from build123d import *

# Parameters (mm, degrees)
SKETCH1_R               = 48.5
SKETCH1_R_2             = 1.5
SKETCH1_W               = 5
SKETCH1_H               = 15
BOSS_EXTRUDE1_DEPTH     = 4
SKETCH1_4_W             = 5
SKETCH1_4_H             = 15
BOSS_EXTRUDE2_DEPTH     = 15
FILLET1_R               = 2
EXTRUDE_THIN1_DEPTH     = 11
SKETCH3_4_R             = 10.5
BOSS_EXTRUDE3_DEPTH     = 11
CUT_EXTRUDE2_DEPTH      = 11
SKETCH8_R               = 1.5
CUT_EXTRUDE3_DEPTH      = 9
SKETCH9_W               = 8
SKETCH9_H               = 4
CUT_EXTRUDE4_DEPTH      = 26
CUT_EXTRUDE4_DEPTH_BACK = 73


with BuildPart() as part:
    # Sketch1 → Boss-Extrude1 (new body)
    with BuildSketch(Plane(origin=(0, 0, 0), x_dir=(1, 0, 0), z_dir=(0, 1, 0))):
        Circle(SKETCH1_R)
        with Locations((7.5, 1.5)):
            Circle(SKETCH1_R_2, mode=Mode.SUBTRACT)
        with Locations((-7.5, 1.5)):
            Circle(SKETCH1_R_2, mode=Mode.SUBTRACT)
        with Locations((-21, -6)):
            Rectangle(SKETCH1_W, SKETCH1_H, mode=Mode.SUBTRACT)
    extrude(amount=BOSS_EXTRUDE1_DEPTH)

    # Sketch1<4> → Boss-Extrude2 (add)
    with BuildSketch(Plane(origin=(0, 0, 0), x_dir=(1, 0, 0), z_dir=(0, 1, 0))):
        with Locations((-21, -6)):
            Rectangle(SKETCH1_4_W, SKETCH1_4_H)
    extrude(amount=BOSS_EXTRUDE2_DEPTH)

    # Fillet1
    fillet1_edges = [part.edges().sort_by_distance(p)[0] for p in [
        (-21, 15, -1.5),
        (-21, 15, 13.5),
    ]]
    fillet(fillet1_edges, radius=FILLET1_R)

    # Sketch3 → Extrude-Thin1 (add, symmetric)
    with BuildSketch(Plane.XY.offset(-16)):
        with BuildLine():
            Line((-33.5, 0), (-33.5, 13.162084514))
            ThreePointArc((-33.5, 13.162084514), (-32.148724822, 19.384006302), (-28.338358569, 24.484924294))
            Line((-28.338358569, 24.484924294), (5.63016077, 54))
            ThreePointArc((5.63016077, 54), (37.663321214, 50.588409815), (31.952020166, 18.884413917))
            ThreePointArc((31.952020166, 18.884413917), (28.210951689, 15.065108917), (26.5, 10))
            Line((26.5, 10), (26.5, 0))
            Line((26.5, 0), (16.5, 0))
            Line((16.5, 0), (16.5, 10.429751474))
            ThreePointArc((16.5, 10.429751474), (19.537286112, 20.046443985), (26.546444335, 27.297484102))
            ThreePointArc((26.546444335, 27.297484102), (29.661699452, 44.590572773), (12.189066483, 46.451440147))
            Line((12.189066483, 46.451440147), (-21.779452856, 16.936364441))
            ThreePointArc((-21.779452856, 16.936364441), (-23.049574941, 15.236058444), (-23.5, 13.162084514))
            Line((-23.5, 13.162084514), (-23.5, 0))
            Line((-23.5, 0), (-33.5, 0))
        make_face()
    extrude(amount=EXTRUDE_THIN1_DEPTH, both=True)

    # Sketch3<4> → Boss-Extrude3 (add)
    with BuildSketch(Plane.XY.offset(-16)):
        with BuildLine():
            Line((-33.5, 0), (-33.5, 13.162084514))
            ThreePointArc((-33.5, 13.162084514), (-32.148724822, 19.384006302), (-28.338358569, 24.484924294))
            Line((-28.338358569, 24.484924294), (5.63016077, 54))
            ThreePointArc((5.63016077, 54), (37.663321214, 50.588409815), (31.952020166, 18.884413917))
            ThreePointArc((31.952020166, 18.884413917), (28.210951689, 15.065108917), (26.5, 10))
            Line((26.5, 10), (26.5, 0))
            Line((26.5, 0), (-33.5, 0))
        make_face()
        with Locations((20.059753337, 37.393168323)):
            Circle(SKETCH3_4_R, mode=Mode.SUBTRACT)
    extrude(amount=BOSS_EXTRUDE3_DEPTH)

    # Sketch5 → Cut-Extrude2 (cut)
    with BuildSketch(Plane(origin=(0, 0, -27), x_dir=(-1, 0, 0), z_dir=(0, 0, -1))):
        with BuildLine():
            Line((-16.5, 4), (25.5, 4))
            ThreePointArc((25.5, 4), (22.632303684, 20.469705569), (12.81364714, 34))
            Line((12.81364714, 34), (-7.597832484, 51.735432044))
            ThreePointArc((-7.597832484, 51.735432044), (-35.262834685, 48.789058703), (-30.330347417, 21.408334972))
            ThreePointArc((-30.330347417, 21.408334972), (-21.973239319, 13.849736754), (-16.5, 4))
        make_face()
    extrude(amount=-CUT_EXTRUDE2_DEPTH, mode=Mode.SUBTRACT)

    # Sketch8 → Cut-Extrude3 (cut)
    with BuildSketch(Plane(origin=(0, 0, -16), x_dir=(-1, 0, 0), z_dir=(0, 0, -1))):
        with Locations((-34.764358033, 43.204760253)):
            Circle(SKETCH8_R)
        with Locations((-28.336481936, 50.865204684)):
            Circle(SKETCH8_R)
        with Locations((8.433651334, 20.011399419)):
            Circle(SKETCH8_R)
        with Locations((2.005775237, 12.350954988)):
            Circle(SKETCH8_R)
        Polygon((-36.322950361, 36.680130765), (-22.181622948, 53.533108514), (9.992243663, 26.536028907), (-4.14908375, 9.683051158), align=None)
    extrude(amount=-CUT_EXTRUDE3_DEPTH, mode=Mode.SUBTRACT)

    # Sketch9 → Cut-Extrude4 (cut, two sides)
    with BuildSketch(Plane.ZY.offset(23.5)) as cut_extrude4_sk:
        with Locations((6, 9)):
            Rectangle(SKETCH9_W, SKETCH9_H)
    extrude(amount=CUT_EXTRUDE4_DEPTH, mode=Mode.SUBTRACT)
    extrude(cut_extrude4_sk.sketch, amount=-CUT_EXTRUDE4_DEPTH_BACK, mode=Mode.SUBTRACT)


solid = part.part
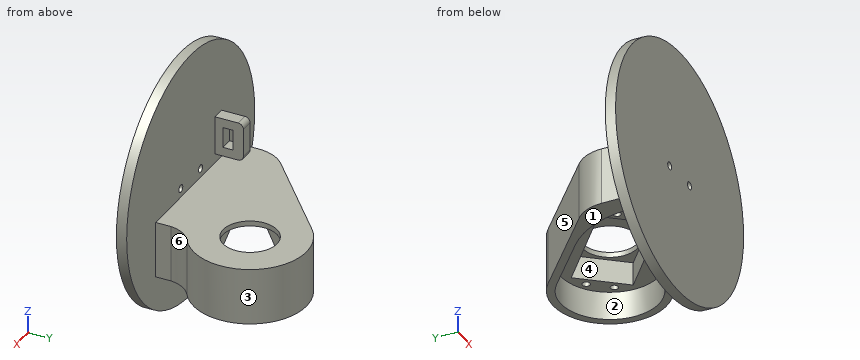
Could you check a few things on this model? Use its own coordinates, in mm. Face numbers are marked on the shaded views. A direction names the side the tool comes from. Give positions to 0.01 mm unless a question says otherwise; leave off trailing zeros. Order: outer loops, then holes, each group sorted by start corner. A loop starts at its lowest first (then second) coordinate and runs counter-clockwise, first axis right, second up. Notation, with made-up numbers: (33.25, 62.5) -> (49.25, 62.5) arc R13 cw to (49.25, 81.5) -> close; hole circle Ø1 at (68.5, -33.5). An arc over 180 degrees is marked (long way). Return JSON: item names as keys, results as strings.
1. Imagine slicing it at A-A on z = -23.5. List the corners of the cut face in (x, y) for me, then the cut area to 3 significant figures.
Answer list:
{"outline": "(-42.43, 0) -> (42.43, 0) -> (42.43, 4) -> (26.5, 4) -> (26.5, 10) arc R12 cw to (31.95, 18.88) arc R22 ccw (long way) to (5.63, 54) -> (-28.34, 24.48) arc R15 ccw to (-33.5, 13.16) -> (-33.5, 4) -> (-42.43, 4) -> close; hole (-25.5, 4) -> (16.5, 4) arc R34.47 cw to (30.33, 21.41) arc R19 ccw (long way) to (7.6, 51.74) -> (-12.81, 34) arc R37.03 ccw to start", "area": "965 mm2"}
2. Imagine slicing it at C-C on z = 40.5. List the corners of the cut face in (x, y) for me.
Answer list:
{"outline": "(-26.68, 0) -> (26.68, 0) -> (26.68, 4) -> (-26.68, 4) -> close"}
3. For pin 1 Ø5 at (x, z) = (-29, -1.5) entering from +Y; pin 2 Ø0.9 at (x, y) = (-2.5, 13) entering from -Z; pin 3 Ø12 at (y, z) = (13, 5) entering from +X, each with a flat end and sliding along its axis, tell me the tip position at first contact or that it passes through.
Answer list:
{"pin 1": "stops at y = 4", "pin 2": "stops at z = -7", "pin 3": "stops at x = -18.5"}
4. Thinking about a two-plate mould opening in X: for the marked faces 1, 2, 3 and 4, which applies, pulls with the +X half, pulls with the -X half, needs draft (parallel to the pull), parting line crosses it, or undercut?
Answer list:
{"face 1": "needs draft", "face 2": "undercut", "face 3": "parting line crosses it", "face 4": "undercut"}
5. I need wall thicknesses on line 1 (X direction, y = 3.1, z = -1.5); line 2 (X direction, y = 3, z = -1); line 3 (Y direction, x = -25.5, z = 13). Which ranges of each line are inside material? Lowest first, please. Write a range as from..to.
Answer list:
{"line 1": "x = -48.48..-9, -6..6, 9..48.48", "line 2": "x = -48.49..-8.91, -6.09..6.09, 8.91..48.49", "line 3": "y = 0..4"}
6. Imagine slicing it at B-B on z = -11. List the corners of the cut face in (x, y) for me, then the cut area to 3 significant figures.
Answer list:
{"outline": "(-47.24, 0) -> (47.24, 0) -> (47.24, 4) -> (26.5, 4) -> (26.5, 10) arc R12 cw to (31.95, 18.88) arc R22 ccw (long way) to (5.63, 54) -> (-28.34, 24.48) arc R15 ccw to (-33.5, 13.16) -> (-33.5, 4) -> (-47.24, 4) -> close; hole (-9.99, 26.54) -> (4.15, 9.68) -> (36.32, 36.68) -> (22.18, 53.53) -> close; hole circle Ø3 at (-8.43, 20.01); hole circle Ø3 at (-2.01, 12.35); hole circle Ø3 at (28.34, 50.87); hole circle Ø3 at (34.76, 43.2)", "area": "2,330 mm2"}
7. On a 3-axis mill with a long thin cutter (end or side, diameter ignored), from which of +Z, -Z, +X, -X, +Y, -Y can I reach the whole of each face in a straight line? I mean the marked faces 5 and 6. Say none if no direction works.
Answer list:
{"face 5": "+Z, -Z, -X, +Y", "face 6": "+Z, -Z, +X"}
